Can you work these out from the drawing? Everything is in mm from the part's minimum corner. Round coordinates to 2 decimals unless told otherwise and drop trailing zeros. Loops run counter-clockwise (first coordinate to the right, second up) from the corner with the lowest first, then second, coordinate; pieces in that order, holes last. Notation, with made-up numbers: (23.5, -26) -> (62.5, -26) arc R24 ccw to (62.5, 4) -> close; hole circle Ø11 at (4, -38.75). An arc over 180 degrees is marked (long way). One line per item, written item: value.
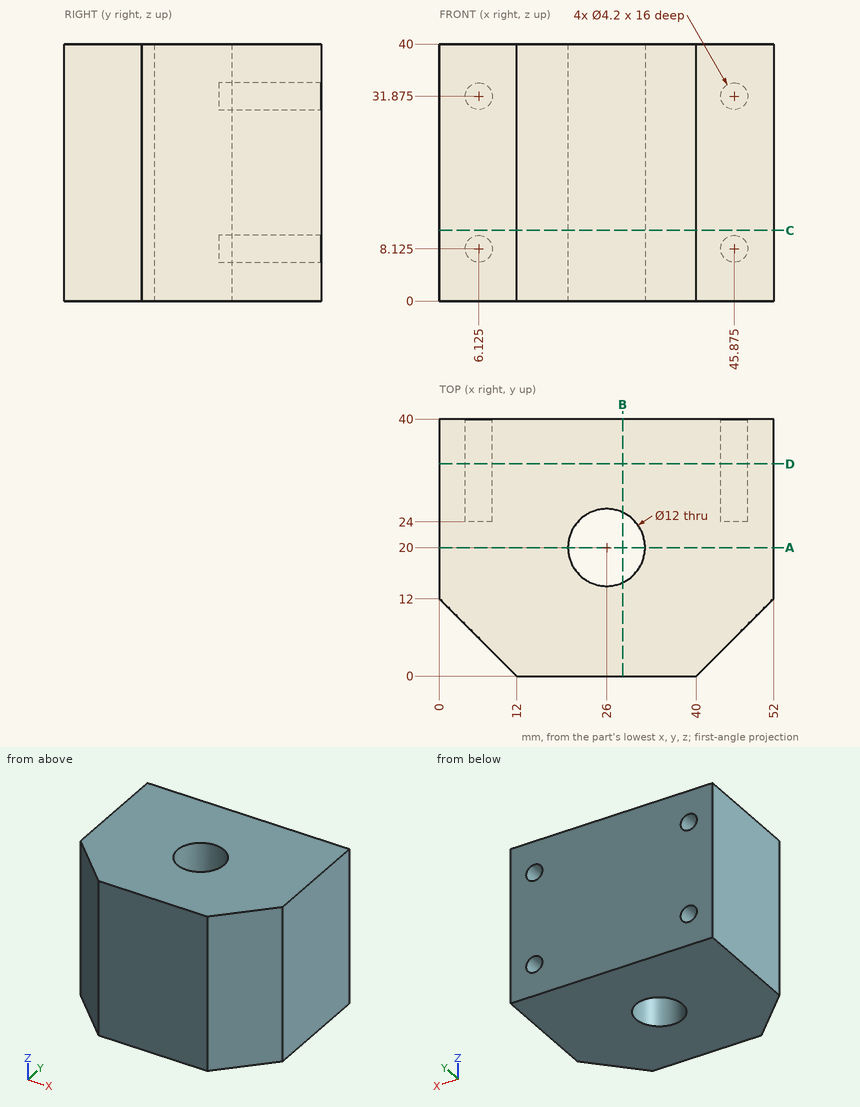
(1) If we section it at A-A, the plane y = 20: Please give me the cut outline in (x, z), then the cut area to 3 significant figures.
Recorded:
outline: (0, 0) -> (20, 0) -> (20, 40) -> (0, 40) -> close; (32, 0) -> (52, 0) -> (52, 40) -> (32, 40) -> close
area: 1,600 mm²
(2) If we section it at D-D, the plane y = 33: Please give me the cut outline in (x, z) (3 decimals).
Recorded:
outline: (0, 0) -> (52, 0) -> (52, 40) -> (0, 40) -> close; hole circle Ø4.2 at (6.125, 8.125); hole circle Ø4.2 at (6.125, 31.875); hole circle Ø4.2 at (45.875, 8.125); hole circle Ø4.2 at (45.875, 31.875)
(3) If we section it at C-C, the plane z = 11: Please give me the cut outline in (x, y), then the cut area to 3 significant figures.
Recorded:
outline: (0, 12) -> (12, 0) -> (40, 0) -> (52, 12) -> (52, 40) -> (0, 40) -> close; hole circle Ø12 at (26, 20)
area: 1,820 mm²
(4) If we section it at B-B, the plane x = 28.5: Please give me the cut outline in (y, z).
Recorded:
outline: (0, 0) -> (14.55, 0) -> (14.55, 40) -> (0, 40) -> close; (25.45, 0) -> (40, 0) -> (40, 40) -> (25.45, 40) -> close
(5) If I drill on L1, parallel to X at y = 17.5, z = 22; L2, parallel to Y at x = 31.5, z = 30; L3, parallel to Y at x = 40.5, z = 11, over which ranges is the centre line in solid material (lowest first)?
Recorded:
L1: 0 to 20.55, 31.45 to 52
L2: 0 to 17.6, 22.4 to 40
L3: 0.5 to 40
(6) I'm going to push flat-ended pins straight in: pin 1 Ø3.5 at (x, z) = (6.125, 31.875) entering from -Y (3 decimals); pin 2 Ø3.5 at (x, z) = (46.5, 7) entering from +Y; pin 3 Ø6.5 at (x, z) = (45.875, 8.125) entering from -Y (3 decimals). Where does each tip first touch, or does it pass through?
Recorded:
pin 1: y = 4.125
pin 2: y = 40
pin 3: y = 2.625
